Verification items for the finished model (mm, model axes). A direction names the side the tool comes from. Coordinates: 2 decimals unless noted, no trailing zeros. Loops run counter-clockwise (first coordinate to the right, second up) from the corner with the lowest first, then second, coordinate; pieces in that order, holes last. Notation, with made-up numbers: (35, 10.5) - (46, 10.5) arc R3 cw to (46, 15.5) - close; hole circle Ø3 at (87.5, -22). An arc over 180 degrees is marked (long way). One line per item, written item: value. Start each with the question number.
(1) Section check B-B (x = 15.5). Record the boundary of the cut face in (y, z), plus the area to 3 significant figures.
(2) Set-up check for faces 4 (the face through (0, 6.5, -6)), 5 (the face through (13.25, 7, -8)), 6 (the face through (17, 7, -10)): record each of +Z, -Z, +X, -X, +Y, -Y from which the full face is reachable in a straight line by a thin tool's end or side.
(3) Draft check along X on faces 1 (the face through (14.5, 7.01, -6.07)), 2 (the face through (20, 1.6, -0.6)), 3 (the face through (-20, 1.6, -0.6)). Enter one of: +X half, -X half, draft (parallel to the pull), parting line (faces both ways), or undercut.
(4) Section check D-D (x = 4). Record the boundary of the cut face in (y, z), plus the area to 3 significant figures.
(5) Section check C-C (z = -6). Record the boundary of the cut face in (x, y), plus the area to 3 significant figures.
(6) Thickness scan on probe 1 along Y at (x, z) = (6.5, -5.25); probe 2 along X at (y, z) = (7.2, -6); probe 3 along Z at (x, y) = (6, 5.5). Record the ranges inside material, lowest first. Write a range as [from, to].
(7) Gauge pin test, flat ends, axial feed: P1, Ø6.5, axis at x = 9, y = -3, coming from the -Z side; P2, Ø4, axis at x = 16, z = -6, coming from the -Y side. Record the tip position at first contact, or that the pin passes through.
(8) Section check A-A (z = -4). Record the boundary of the cut face in (x, y), plus the area to 3 significant figures.
```python
from build123d import *

# Parameters (mm, degrees)
SZKIC1_W                           = 40
SZKIC1_H                           = 15
ODGI_CIE_BAZOWE1_DEPTH             = 1
ODGI_CIE_KRAW_DZI1_STRIP_W         = 5.4732
ODGI_CIE_KRAW_DZI1_STRIP_H         = 1
ODGI_CIE_KRAW_DZI1_STRIP_CUT_DEPTH = 40
ODGI_CIE_KRAW_DZI1_DEPTH           = 40
OTW_R_GWINTOWANY_M3X0_51_D         = 2.5
WYTNIJ_WYCI_GNI_CIE1_DEPTH         = 27.381811917
OTWORY_USTALAJ_CE_3_0MM1_D         = 3


# Sheet-metal steps are written as plain solids
with BuildPart() as part:
    # Szkic1 → Odgięcie bazowe1 (new body)
    with BuildSketch(Plane.XY):
        Rectangle(SZKIC1_W, SZKIC1_H)
    extrude(amount=-ODGI_CIE_BAZOWE1_DEPTH)

    # Odgięcie krawędzi1 strip (across the edge) → Odgięcie krawędzi1 strip cut (cut)
    with BuildSketch(Plane(origin=(-20, 7.5, -1), x_dir=(0, -1, 0), z_dir=(1, 0, 0))):
        with Locations((-1, -0.5)):
            Rectangle(ODGI_CIE_KRAW_DZI1_STRIP_W, ODGI_CIE_KRAW_DZI1_STRIP_H)
    extrude(amount=ODGI_CIE_KRAW_DZI1_STRIP_CUT_DEPTH, mode=Mode.SUBTRACT)

    # Odgięcie krawędzi1 section (across the edge) → Odgięcie krawędzi1 (add)
    with BuildSketch(Plane(origin=(-20, 7.5, -1), x_dir=(0, -1, 0), z_dir=(1, 0, 0))):
        with BuildLine():
            Line((0, 0.7366), (0, 9))
            Line((0, 9), (1, 9))
            Line((1, 9), (1, 0.7366))
            ThreePointArc((1, 0.7366), (1.215745145, 0.215745145), (1.7366, 0))
            Line((1.7366, 0), (1.7366, -1))
            ThreePointArc((1.7366, -1), (0.508638364, -0.491361636), (0, 0.7366))
        make_face()
    extrude(amount=ODGI_CIE_KRAW_DZI1_DEPTH)

    # Otwór gwintowany M3x0.51 (through all)
    with Locations(Plane.XY):
        with Locations((-9, -1.5), (9, -1.5)):
            Hole(OTW_R_GWINTOWANY_M3X0_51_D / 2)

    # Szkic11 → Wytnij-wyciągnięcie1 (cut, through all)
    with BuildSketch(Plane.XZ.offset(-6.5)):
        with BuildLine():
            ThreePointArc((-10.567890835, -10), (-12.490797584, -8.887684697), (-13.25, -6.8))
            Line((-13.25, -6.8), (-13.25, -10))
            Line((-13.25, -10), (-10.567890835, -10))
        make_face()
        with BuildLine():
            Line((-6.75, -10), (-6.75, -6.8))
            ThreePointArc((-6.75, -6.8), (-7.509202416, -8.887684697), (-9.432109165, -10))
            Line((-9.432109165, -10), (-6.75, -10))
        make_face()
        with BuildLine():
            ThreePointArc((-6.75, -6.8), (-10, -3.55), (-13.25, -6.8))
            ThreePointArc((-13.25, -6.8), (-12.490797584, -8.887684697), (-10.567890835, -10))
            Line((-10.567890835, -10), (-9.432109165, -10))
            ThreePointArc((-9.432109165, -10), (-7.509202416, -8.887684697), (-6.75, -6.8))
        make_face()
        with BuildLine():
            Line((-9.432109165, -10), (-10.567890835, -10))
            ThreePointArc((-10.567890835, -10), (-10, -10.05), (-9.432109165, -10))
        make_face()
        with BuildLine():
            ThreePointArc((13.25, -6.8), (10, -3.55), (6.75, -6.8))
            ThreePointArc((6.75, -6.8), (7.509202416, -8.887684697), (9.432109165, -10))
            Line((9.432109165, -10), (10.567890835, -10))
            ThreePointArc((10.567890835, -10), (12.490797584, -8.887684697), (13.25, -6.8))
        make_face()
        with BuildLine():
            Line((10.567890835, -10), (9.432109165, -10))
            ThreePointArc((9.432109165, -10), (10, -10.05), (10.567890835, -10))
        make_face()
        with BuildLine():
            Line((6.75, -6.8), (6.75, -10))
            Line((6.75, -10), (9.432109165, -10))
            ThreePointArc((9.432109165, -10), (7.509202416, -8.887684697), (6.75, -6.8))
        make_face()
        with BuildLine():
            Line((13.25, -10), (13.25, -6.8))
            ThreePointArc((13.25, -6.8), (12.490797584, -8.887684697), (10.567890835, -10))
            Line((10.567890835, -10), (13.25, -10))
        make_face()
    extrude(amount=-WYTNIJ_WYCI_GNI_CIE1_DEPTH, mode=Mode.SUBTRACT)

    # Otwory ustalające Ø3.0mm1 (through all)
    with Locations(Plane(origin=(0, 6.5, 0), x_dir=(-1, 0, 0), z_dir=(0, -1, 0))):
        with Locations((16, 6), (-16, 6)):
            Hole(OTWORY_USTALAJ_CE_3_0MM1_D / 2)


solid = part.part
```
Responses:
1. outline: (-7.5, -1) - (5.76, -1) arc R0.74 cw to (6.5, -1.74) - (6.5, -4.59) - (7.5, -4.59) - (7.5, -1.74) arc R1.74 ccw to (5.76, 0) - (-7.5, 0) - close; (6.5, -10) - (7.5, -10) - (7.5, -7.41) - (6.5, -7.41) - close
1. area: 20.6 mm²
2. face 4: -Z, +X, -X, -Y
2. face 5: -Z, +Y, -Y
2. face 6: -Z, +X, -X, +Y, -Y
3. face 1: undercut
3. face 2: +X half
3. face 3: -X half
4. outline: (-7.5, -1) - (5.76, -1) arc R0.74 cw to (6.5, -1.74) - (6.5, -10) - (7.5, -10) - (7.5, -1.74) arc R1.74 ccw to (5.76, 0) - (-7.5, 0) - close
4. area: 23.5 mm²
5. outline: (-20, 6.5) - (-17.5, 6.5) - (-17.5, 7.5) - (-20, 7.5) - close; (-14.5, 6.5) - (-13.15, 6.5) - (-13.15, 7.5) - (-14.5, 7.5) - close; (-6.85, 6.5) - (6.85, 6.5) - (6.85, 7.5) - (-6.85, 7.5) - close; (13.15, 6.5) - (14.5, 6.5) - (14.5, 7.5) - (13.15, 7.5) - close; (17.5, 6.5) - (20, 6.5) - (20, 7.5) - (17.5, 7.5) - close
5. area: 21.4 mm²
6. probe 1: y = [6.5, 7.5]
6. probe 2: x = [-20, -17.5], [-14.5, -13.15], [-6.85, 6.85], [13.15, 14.5], [17.5, 20]
6. probe 3: z = [-1, 0]
7. P1: stops at z = -1
7. P2: stops at y = 6.5
8. outline: (-20, 6.5) - (-11.65, 6.5) - (-11.65, 7.5) - (-20, 7.5) - close; (-8.35, 6.5) - (8.35, 6.5) - (8.35, 7.5) - (-8.35, 7.5) - close; (11.65, 6.5) - (20, 6.5) - (20, 7.5) - (11.65, 7.5) - close
8. area: 33.4 mm²
